Build history of the part. All positions in model axes, mm. Give positions to 0.01 mm unless a question says otherwise; leave off trailing zeros. One line per question, with ' | ' between items. Start each with the question number.
(1) Drill centre lines: probe 1 along X at (y, z) = (0.15, -6.5); probe 2 along Z at (x, y) = (-132, 0.1); probe 3 along X at (y, z) = (0.1, -3.5). Where is each one in solid material? Low to high. Write a range as from..to.
(2) Pull direction Z, two halves, no side cores. Call faces 1 (the flat face through (-2, 1.016, -1)), 2 (the cylindrical face through (-69.123, 0.501, -6.022)), 3 (the cylindrical face through (136.02, 0.5, -52.08)): released by +Z, released by -Z, zero draft, split by the parting line, or undercut.
(3) Pin check, flat tip, straight feed: P1, Ø9, axis at x = -132.17, z = -51.03, coming from the +Y side. Stop position of the tip, or through.
from build123d import *

# Parameters (mm, degrees)
CROQUIS1_W              = 300.0502
CROQUIS1_H              = 115.8748
CROQUIS1_R              = 3.5052
SALIENTE_EXTRUIR1_DEPTH = 1.016


with BuildPart() as part:
    # Croquis1 → Saliente-Extruir1 (new body)
    with BuildSketch(Plane(origin=(0, 0, 0), x_dir=(1, 0, 0), z_dir=(0, 1, 0))):
        Rectangle(CROQUIS1_W, CROQUIS1_H)
        with Locations((-128.1049, -52.0446)):
            Circle(CROQUIS1_R, mode=Mode.SUBTRACT)
        with Locations((-132.1689, 51.0286)):
            Circle(CROQUIS1_R, mode=Mode.SUBTRACT)
        with Locations((-10.5791, 51.0286)):
            Circle(CROQUIS1_R, mode=Mode.SUBTRACT)
        with Locations((132.6769, 51.0286)):
            Circle(CROQUIS1_R, mode=Mode.SUBTRACT)
        with Locations((132.6769, -52.0446)):
            Circle(CROQUIS1_R, mode=Mode.SUBTRACT)
        with Locations((-29.2989, -52.0446)):
            Circle(CROQUIS1_R, mode=Mode.SUBTRACT)
        with Locations((67.9069, 5.8674)):
            Circle(CROQUIS1_R, mode=Mode.SUBTRACT)
        with Locations((-65.6209, 5.8674)):
            Circle(CROQUIS1_R, mode=Mode.SUBTRACT)
    extrude(amount=SALIENTE_EXTRUIR1_DEPTH)


solid = part.part
Results:
1) probe 1: x = -150.03..-69.07, -62.17..64.46, 71.35..150.03 | probe 2: z = -57.94..-54.53, -47.53..57.94 | probe 3: x = -150.03..-68.21, -63.04..65.32, 70.49..150.03
2) face 1: zero draft | face 2: undercut | face 3: undercut
3) P1: stops at y = 1.02
